Answer from the drawing. Dimensions are ordinates in mm from the lowest x, y and z of the part. Coordinates: 2 decimals unless noted, no trailing zeros. Order: outer loops, then holes, each group sorted by start corner. A loop starts at its lowest first (then second) coordinate and runs counter-clockwise, first axis right, second up. Notation, with made-up numbers: (85.5, 46) - (134.5, 46) arc R24 cw to (134.5, 62) - close; hole circle Ø4 at (3.5, 86). An arc over 180 degrees is marked (long way). Use a Markdown table: item, result. Add a question column.
Item 1: The part is cut by section B-B, the plane y = 3.5. Give the vertices of the cut face in (x, z).
Item 2: Flat-ended cylindrical pins translate along their axes: P1, Ø2, axis at x = 137.3, y = 7.28, coming from the -Z side; P2, Ø4, axis at x = 21, z = 3.5, coming from the +Y side; P3, Ø4, axis at x = 90.5, z = 3, coming from the -Y side (1 decimal); P4, Ø5, axis at x = 59.5, y = 10, coming from the -Z side. Find the tip coordinate at first contact, or state that the pin passes through.
Item 3: The part is cut by section D-D, the plane y = 11.5. Give the vertices of the cut face in (x, z), then the cut area to 3 significant figures.
Item 4: Find the intervals of material crossed by line 1 along Y through (x, z) = (19.5, 7.5); line 2 along X through (y, z) = (6.25, 11.5), in increasing order.
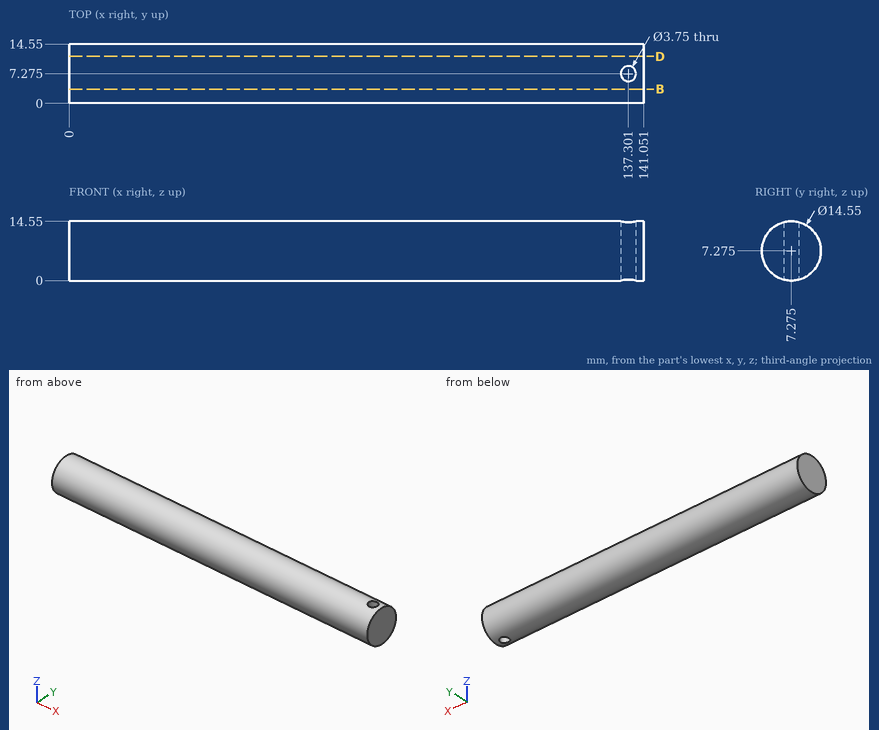
Solution:
| question | item | result |
|---|---|---|
| 1 | outline | (0, 1.06) - (141.05, 1.06) - (141.05, 13.49) - (0, 13.49) - close |
| 2 | P1 | passes through |
| 2 | P2 | stops at y = 14.33 |
| 2 | P3 | stops at y = 0.4 |
| 2 | P4 | stops at z = 0 |
| 3 | outline | (0, 1.35) - (141.05, 1.35) - (141.05, 13.2) - (0, 13.2) - close |
| 3 | area | 1,670 mm2 |
| 4 | line 1 | y = 0 to 14.55 |
| 4 | line 2 | x = 0 to 135.73, 138.87 to 141.05 |
